Autodesk Inventor part; units mm, degrees
ref_plane "YZ Plane" through (0, 0, 0) normal (1, 0, 0) x (0, 1, 0)
ref_plane "XZ Plane" through (0, 0, 0) normal (0, 1, 0) x (-1, 0, 0)
ref_plane "XY Plane" through (0, 0, 0) normal (0, 0, 1) x (1, 0, 0)
ref_plane "Work Plane1" through (0, 0, 0) normal (0, 0, 1) x (1, 0, 0)
sketch "Sketch1" plane through (0, 0, 0) normal (0, 0, 1) x (1, 0, 0)
  circle A0 centre (-0.1312, 6.3486) radius 1.5875
  circle A1 centre (6.3486, 0.1312) radius 1.5875
  circle A2 centre (0.1312, -6.3486) radius 1.5875
  circle A3 centre (-6.3486, -0.1312) radius 1.5875
  arc A4 (-1.8, 2.4) -> (1.8, 2.4) centre (0, 0) ccw
  arc A5 (-10.2062, 24.6399) -> (-9.5905, 18.6316) centre (10.2722, 23.7027) ccw
  arc A6 (-9.5905, 18.6316) -> (-11.0963, 17.7759) centre (0, 0) ccw
  arc A7 (-11.0963, 17.7759) -> (-15.9426, 21.3804) centre (-25.6201, 3.3086) ccw
  arc A8 (-15.9426, 21.3804) -> (-17.6537, 19.9909) centre (0, 0) ccw
  arc A9 (-17.6537, 19.9909) -> (-15.1205, 14.508) centre (2.0194, 25.7538) ccw
  arc A10 (-15.1205, 14.508) -> (-16.2669, 13.2098) centre (0, 0) ccw
  arc A11 (-16.2669, 13.2098) -> (-22.021, 15.0454) centre (-25.3062, -5.1895) ccw
  arc A12 (-22.021, 15.0454) -> (-23.1882, 13.1756) centre (0, 0) ccw
  arc A13 (-23.1882, 13.1756) -> (-19.012, 8.8123) centre (-6.4522, 25.0141) ccw
  arc A14 (-19.012, 8.8123) -> (-19.6747, 7.2122) centre (0, 0) ccw
  arc A15 (-19.6747, 7.2122) -> (-25.7131, 7.08) centre (-22.2501, -13.1252) ccw
  arc A16 (-25.7131, 7.08) -> (-26.2099, 4.9325) centre (0, 0) ccw
  arc A17 (-26.2099, 4.9325) -> (-20.8432, 2.1617) centre (-14.2247, 21.5637) ccw
  arc A18 (-20.8432, 2.1617) -> (-20.9505, 0.4331) centre (0, 0) ccw
  arc A19 (-20.9505, 0.4331) -> (-26.6187, -1.6526) centre (-16.7827, -19.6386) ccw
  arc A20 (-26.6187, -1.6526) -> (-26.3914, -3.8451) centre (0, 0) ccw
  arc A21 (-26.3914, -3.8451) -> (-20.4158, -4.7232) centre (-20.4557, 15.7766) ccw
  arc A22 (-20.4158, -4.7232) -> (-19.956, -6.393) centre (0, 0) ccw
  arc A23 (-19.956, -6.393) -> (-24.6399, -10.2062) centre (-9.4967, -24.0239) ccw
  arc A24 (-24.6399, -10.2062) -> (-23.7129, -12.2061) centre (0, 0) ccw
  arc A25 (-23.7129, -12.2061) -> (-17.7759, -11.0963) centre (-24.47, 8.2798) ccw
  arc A26 (-17.7759, -11.0963) -> (-16.7989, -12.5263) centre (0, 0) ccw
  arc A27 (-16.7989, -12.5263) -> (-19.9909, -17.6537) centre (-1.1816, -25.8058) ccw
  arc A28 (-19.9909, -17.6537) -> (-18.4648, -19.2443) centre (0, 0) ccw
  arc A29 (-18.4648, -19.2443) -> (-13.2098, -16.2669) centre (-25.8326, -0.1142) ccw
  arc A30 (-13.2098, -16.2669) -> (-11.8214, -17.3022) centre (0, 0) ccw
  arc A31 (-11.8214, -17.3022) -> (-13.1756, -23.1882) centre (7.2615, -24.7913) ccw
  arc A32 (-13.1756, -23.1882) -> (-11.2157, -24.197) centre (0, 0) ccw
  arc A33 (-11.2157, -24.197) -> (-7.2122, -19.6747) centre (-24.3958, -8.4958) ccw
  arc A34 (-7.2122, -19.6747) -> (-5.5629, -20.2031) centre (0, 0) ccw
  arc A35 (-5.5629, -20.2031) -> (-4.9325, -26.2099) centre (14.9178, -21.0902) ccw
  arc A36 (-4.9325, -26.2099) -> (-2.7512, -26.5277) centre (0, 0) ccw
  arc A37 (-2.7512, -26.5277) -> (-0.4331, -20.9505) centre (-20.3154, -15.9568) ccw
  arc A38 (-0.4331, -20.9505) -> (1.2985, -20.9147) centre (0, 0) ccw
  arc A39 (1.2985, -20.9147) -> (3.8451, -26.3914) centre (20.9575, -15.1037) ccw
  arc A40 (3.8451, -26.3914) -> (6.0114, -25.9837) centre (0, 0) ccw
  arc A41 (6.0114, -25.9837) -> (6.393, -19.956) centre (-14.0335, -21.6886) ccw
  arc A42 (6.393, -19.956) -> (8.0191, -19.3599) centre (0, 0) ccw
  arc A43 (8.0191, -19.3599) -> (12.2061, -23.7129) centre (24.7261, -7.4804) ccw
  arc A44 (12.2061, -23.7129) -> (14.1226, -22.6239) centre (0, 0) ccw
  arc A45 (14.1226, -22.6239) -> (12.5263, -16.7989) centre (-6.2308, -25.0702) ccw
  arc A46 (12.5263, -16.7989) -> (13.8708, -15.7071) centre (0, 0) ccw
  arc A47 (13.8708, -15.7071) -> (19.2443, -18.4648) centre (25.8152, 0.9534) ccw
  arc A48 (19.2443, -18.4648) -> (20.7033, -16.8125) centre (0, 0) ccw
  arc A49 (20.7033, -16.8125) -> (17.3022, -11.8214) centre (2.2471, -25.7349) ccw
  arc A50 (17.3022, -11.8214) -> (18.2193, -10.3522) centre (0, 0) ccw
  arc A51 (18.2193, -10.3522) -> (24.197, -11.2157) centre (24.1069, 9.284) ccw
  arc A52 (24.197, -11.2157) -> (25.0406, -9.1792) centre (0, 0) ccw
  arc A53 (25.0406, -9.1792) -> (20.2031, -5.5629) centre (10.4814, -23.6109) ccw
  arc A54 (20.2031, -5.5629) -> (20.5935, -3.8755) centre (0, 0) ccw
  arc A55 (20.5935, -3.8755) -> (26.5277, -2.7512) centre (19.7863, 16.6084) ccw
  arc A56 (26.5277, -2.7512) -> (26.6643, -0.5512) centre (0, 0) ccw
  arc A57 (26.6643, -0.5512) -> (20.9147, 1.2985) centre (17.58, -18.9283) ccw
  arc A58 (20.9147, 1.2985) -> (20.7361, 3.0212) centre (0, 0) ccw
  arc A59 (20.7361, 3.0212) -> (25.9837, 6.0114) centre (13.3214, 22.1331) ccw
  arc A60 (25.9837, 6.0114) -> (25.3985, 8.1366) centre (0, 0) ccw
  arc A61 (25.3985, 8.1366) -> (19.3599, 8.0191) centre (22.7734, -12.1945) ccw
  arc A62 (19.3599, 8.0191) -> (18.6316, 9.5905) centre (0, 0) ccw
  arc A63 (18.6316, 9.5905) -> (22.6239, 14.1226) centre (5.413, 25.2594) ccw
  arc A64 (22.6239, 14.1226) -> (21.3804, 15.9426) centre (0, 0) ccw
  arc A65 (21.3804, 15.9426) -> (15.7071, 13.8708) centre (25.4991, -4.1393) ccw
  arc A66 (15.7071, 13.8708) -> (14.508, 15.1205) centre (0, 0) ccw
  arc A67 (14.508, 15.1205) -> (16.8125, 20.7033) centre (-3.082, 25.6483) ccw
  arc A68 (16.8125, 20.7033) -> (15.0454, 22.021) centre (0, 0) ccw
  arc A69 (15.0454, 22.021) -> (10.3522, 18.2193) centre (25.4615, 4.3646) ccw
  arc A70 (10.3522, 18.2193) -> (8.8123, 19.012) centre (0, 0) ccw
  arc A71 (8.8123, 19.012) -> (9.1792, 25.0406) centre (-11.243, 23.2579) ccw
  arc A72 (9.1792, 25.0406) -> (7.08, 25.7131) centre (0, 0) ccw
  arc A73 (7.08, 25.7131) -> (3.8755, 20.5935) centre (22.6647, 12.3954) ccw
  arc A74 (3.8755, 20.5935) -> (2.1617, 20.8432) centre (0, 0) ccw
  arc A75 (2.1617, 20.8432) -> (0.5512, 26.6643) centre (-18.1856, 18.3472) ccw
  arc A76 (0.5512, 26.6643) -> (-1.6526, 26.6187) centre (0, 0) ccw
  arc A77 (-1.6526, 26.6187) -> (-3.0212, 20.7361) centre (17.4119, 19.083) ccw
  arc A78 (-3.0212, 20.7361) -> (-4.7232, 20.4158) centre (0, 0) ccw
  arc A79 (-4.7232, 20.4158) -> (-8.1366, 25.3985) centre (-23.1576, 11.4482) ccw
  arc A80 (-8.1366, 25.3985) -> (-10.2062, 24.6399) centre (0, 0) ccw
  circle A81 centre (0, 0) radius 34.925
  line L0 (-3.1504, 2.4) -> (-1.8, 2.4)
  line L1 (1.8, 2.4) -> (3.3261, 2.4)
  line L2 (-1.8, 2.4) -> (1.8, 2.4)
  point P0 (0.0879, -3)
  dimension "d0" = 69.85
  dimension "d3" = 6
  dimension "d4" = 5.4
extrude "Extrusion1" add sketch "Sketch1" along normal blind 3.175 contours A80 A79 A78 A77 A76 A75 A74 A73 A72 A71 A70 A69 A68 A67 A66 A65 A64 A63 A62 A61 A60 A59 A58 A57 A56 A55 A54 A53 A52 A51 A50 A49 A48 A47 A46 A45 A44 A43 A42 A41 A40 A39 A38 A37 A36 A35 A34 A33 A32 A31 A30 A29 A28 A27 A26 A25 A24 A23 A22 A21 A20 A19 A18 A17 A16 A15 A14 A13 A12 A11 A10 A9 A8 A7 A6 A5 | A81
properties part number "gearGuideRings"
Build history of the part. All positions in model axes, mm. A direction names the side the tool comes from. Round coordinates to 2 decimals unless told otherwise and drop trailing zeros. Write each loop counter-clockwise with the first axis right and the second up, starting at its lowest first coordinate (ties: lowest second). Pieces come first, ordered by that corner, then holes. Notation, with made-up numbers: (-5.5, 82) - (39.5, 82) arc R12 ccw to (39.5, 86) - close; hole circle Ø6 at (12.25, 17.5). An arc over 180 degrees is marked (long way). Write each question's results on one line, items separated by ' | '. Start each with the question number.
Item 1: Saw through at A-A (x = 0). Write the cut outline in (y, z) (3 decimals).
Item 2: Which spindle directions (+Z, -Z, +X, -X, +Y, -Y) get a long thin tool onto all of the face, cutting with end or side? Do faces 1 (the face through (-0.5, 8.3, 3.175)), 2 (the face through (0, 2.4, 2)). Say none if no direction does.
Item 3: Mould opens along X. For faces 3 (the face through (-27.715, 21.251, 1.565)), 4 (the face through (-0.5, 8.3, 0)), 5 (the face through (0.72, 5.01, 1.57)) say: pulls with the +X half, pulls with the -X half, needs draft (parallel to the pull), parting line crosses it, or undercut.
Item 4: Drop flat-ended pins along their axis: P1, Ø1.5, axis at x = 18.5, z = 1.5, coming from the +Y side; P2, Ø1.6, axis at x = -0.5, z = 1, coming from the -Y side (3 decimals). Give the stop position or say it passes through.
Item 5: Wall check: L1, parallel to X at y = -1, z = 0.8; L2, parallel to X at y = 2, z = 1.05; L3, parallel to Y at x = -7.5, z = 2.3. Give the ranges that are in metal, low to high. Write a range as [from, to].
Item 6: Saw through at D-D (x = 9). Write the cut outline in (y, z) (3 decimals), and give its area (3 significant figures).
Item 7: Saw through at B-B (z = 1.95). State how many separate pieces and enclosed holes the cut face has, and give its area (3 significant figures).
Item 8: Saw through at C-C (y = 29.5). Write the cut outline in (x, z) (3 decimals), and give its area (3 significant figures).
Results are:
1) outline: (-34.925, 0) - (-7.931, 0) - (-7.931, 3.175) - (-34.925, 3.175) - close; (-4.767, 0) - (-3, 0) - (-3, 3.175) - (-4.767, 3.175) - close; (2.4, 0) - (4.767, 0) - (4.767, 3.175) - (2.4, 3.175) - close; (7.931, 0) - (34.925, 0) - (34.925, 3.175) - (7.931, 3.175) - close
2) face 1: +Z, +X, -X, +Y, -Y | face 2: +Z, -Z
3) face 3: parting line crosses it | face 4: needs draft | face 5: undercut
4) P1: stops at y = 30.08 | P2: stops at y = -34.925
5) L1: x = [-34.91, -7.68], [-5.02, -2.83], [2.83, 5.23], [7.46, 34.91] | L2: x = [-34.87, -2.24], [2.24, 34.87] | L3: y = [-34.11, -1.22], [0.96, 34.11]
6) outline: (-33.745, 0) - (33.745, 0) - (33.745, 3.175) - (-33.745, 3.175) - close | area: 214 mm²
7) separate pieces: 1 | enclosed holes: 5 | area: 3,770 mm²
8) outline: (-18.695, 0) - (18.695, 0) - (18.695, 3.175) - (-18.695, 3.175) - close | area: 119 mm²
